Read the model definition and answer for the solid it produces. Units are mm, in the model's axes. Face numbers are marked on the shaded views. A direction names the side the tool comes from. Round coordinates to 2 decimals unless told otherwise and drop trailing zeros. Order: outer loops, then holes, each group sorted by start corner. A loop starts at its lowest first (then second) coordinate and runs counter-clockwise, first axis right, second up. Notation, with made-up numbers: (76, 27.25) - (105, 27.25) arc R26 ccw to (105, 41.25) - close; hole circle Ø5 at (11, 32). An arc over 180 degrees is marked (long way). Put each result on its own line as item: value. Start each with the question number.
Q1. Which of the six approach directions +Z, -Z, +X, -X, +Y, -Y give full straight-line access (tool end or side, diameter ignored) to the marked faces 1 and 2?
Q2. Section C-C on y = 304.5 is taken. Give the vertices of the cut face in (x, z).
Q3. Section A-A on z = 4.25 is taken. Give the vertices of the cut face in (x, y) (3 decimals).
Q4. This flat-tipped pin is pushed along its axis until it touches: pin 1 Ø3 at (x, z) = (12, -10) entering from +Y. Where does it stop, or does it pass through?
Q5. Find the intervals of material crossed by line 1 along Z through (x, y) = (1, 251); line 2 along X through (y, z) = (269.5, -9), in increasing order. Write a range as from..to.
Q6. Section B-B on x = -15.5 is taken. Give the vertices of the cut face in (y, z) (3 decimals), then the cut area to 3 significant figures.
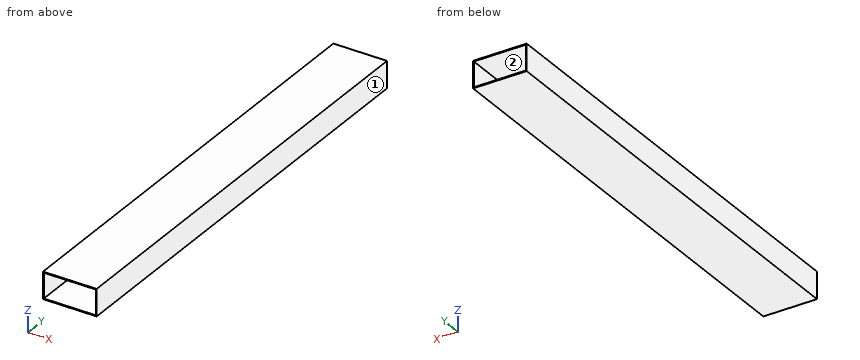
from build123d import *

# Parameters (mm, degrees)
SKETCH1_W           = 50.8
SKETCH1_H           = 25.4
BOSS_EXTRUDE1_DEPTH = 762
SKETCH2_W           = 49.1998
SKETCH2_H           = 23.7998
CUT_EXTRUDE1_DEPTH  = 763.528983056
SKETCH3_W           = 50.8
SKETCH3_H           = 25.4
CUT_EXTRUDE2_DEPTH  = 333.375


with BuildPart() as part:
    # Sketch1 → Boss-Extrude1 (new body)
    with BuildSketch(Plane(origin=(0, 0, 0), x_dir=(1, 0, 0), z_dir=(0, 1, 0))):
        Rectangle(SKETCH1_W, SKETCH1_H)
    extrude(amount=BOSS_EXTRUDE1_DEPTH)

    # Sketch2 → Cut-Extrude1 (cut, through all)
    with BuildSketch(Plane.XZ):
        Rectangle(SKETCH2_W, SKETCH2_H)
    extrude(amount=-CUT_EXTRUDE1_DEPTH, mode=Mode.SUBTRACT)

    # Sketch3 → Cut-Extrude2 (cut)
    with BuildSketch(Plane(origin=(0, 762, 0), x_dir=(1, 0, 0), z_dir=(0, 1, 0))):
        Rectangle(SKETCH3_W, SKETCH3_H)
    extrude(amount=-CUT_EXTRUDE2_DEPTH, mode=Mode.SUBTRACT)


solid = part.part
Findings:
1. face 1: +Z, -Z, +X, +Y, -Y
1. face 2: +Y, -Y
2. outline: (-25.4, -12.7) - (25.4, -12.7) - (25.4, 12.7) - (-25.4, 12.7) - close; hole (-24.6, -11.9) - (24.6, -11.9) - (24.6, 11.9) - (-24.6, 11.9) - close
3. outline: (-25.4, 0) - (-24.6, 0) - (-24.6, 428.625) - (-25.4, 428.625) - close; (24.6, 0) - (25.4, 0) - (25.4, 428.625) - (24.6, 428.625) - close
4. pin 1: through
5. line 1: -12.7..-11.9, 11.9..12.7
5. line 2: -25.4..-24.6, 24.6..25.4
6. outline: (0, -12.7) - (428.625, -12.7) - (428.625, -11.9) - (0, -11.9) - close; (0, 11.9) - (428.625, 11.9) - (428.625, 12.7) - (0, 12.7) - close
6. area: 686 mm2
